Design review of the part built by this model. Coordinates are the model's own, in mm. Coordinates: 2 decimals unless noted, no trailing zeros. Order: outer loops, then holes, each group sorted by start corner. A loop starts at its lowest first (then second) coordinate and runs counter-clockwise, first axis right, second up. Notation, with made-up numbers: M 24.5,-32.75 L 69.5,-32.75 A18 ccw 69.5,-27.75 Z; hole C -35.5,11 d3. An arc over 180 degrees is marked long. Answer as a JSON object with one key per item and string values.
Autodesk Inventor part; units mm, degrees
ref_plane "YZ Plane" through (0, 0, 0) normal (1, 0, 0) x (0, 1, 0)
ref_plane "XZ Plane" through (0, 0, 0) normal (0, 1, 0) x (-1, 0, 0)
ref_plane "XY Plane" through (0, 0, 0) normal (0, 0, 1) x (1, 0, 0)
sketch "Sketch1" plane through (0, 0, 0) normal (0, 0, 1) x (1, 0, 0)
  line L0 (-37.6936, 53.8926) -> (212.3064, 53.8926)
  line L1 (212.3064, 53.8926) -> (212.3064, -66.1074)
  line L2 (212.3064, -66.1074) -> (-37.6936, -66.1074)
  line L3 (-37.6936, -66.1074) -> (-37.6936, 53.8926)
  line L4 (12.3064, -66.1074) -> (162.3064, -66.1074)
  line L5 (162.3064, -66.1074) -> (162.3064, 3.8926)
  line L6 (162.3064, 3.8926) -> (12.3064, 3.8926)
  line L7 (12.3064, 3.8926) -> (12.3064, -66.1074)
  line L8 (-37.6936, 53.8926) -> (-34.6936, 53.8926)
  line L9 (-34.6936, 53.8926) -> (-34.6936, 33.8926)
  line L10 (-34.6936, 33.8926) -> (-37.6936, 33.8926)
  line L11 (-37.6936, 33.8926) -> (-37.6936, 53.8926)
  line L12 (-37.6936, 33.8926) -> (-34.6936, 33.8926)
  line L13 (-34.6936, 33.8926) -> (-34.6936, 13.9926)
  line L14 (-34.6936, 13.9926) -> (-37.6936, 13.9926)
  line L15 (-37.6936, 13.9926) -> (-37.6936, 33.8926)
  line L16 (-37.6936, 13.9926) -> (-34.6936, 13.9926)
  line L17 (-34.6936, 13.9926) -> (-34.6936, -6.0074)
  line L18 (-34.6936, -6.0074) -> (-37.6936, -6.0074)
  line L19 (-37.6936, -6.0074) -> (-37.6936, 13.9926)
  line L20 (-34.6936, -6.0074) -> (-37.6936, -6.0074)
  line L21 (-37.6936, -6.0074) -> (-37.6936, -25.9074)
  line L22 (-37.6936, -25.9074) -> (-34.6936, -25.9074)
  line L23 (-34.6936, -25.9074) -> (-34.6936, -6.0074)
  line L24 (-37.6936, -25.9074) -> (-34.6936, -25.9074)
  line L25 (-34.6936, -25.9074) -> (-34.6936, -45.9074)
  line L26 (-34.6936, -45.9074) -> (-37.6936, -45.9074)
  line L27 (-37.6936, -45.9074) -> (-37.6936, -25.9074)
  line L28 (-34.6936, -45.9074) -> (-37.6936, -45.9074)
  line L29 (-37.6936, -45.9074) -> (-37.6936, -66.1074)
  line L30 (-37.6936, -66.1074) -> (-34.6936, -66.1074)
  line L31 (-34.6936, -66.1074) -> (-34.6936, -45.9074)
  line L32 (212.3064, -66.1074) -> (212.3064, 53.8926)
  line L33 (212.3064, 53.8926) -> (209.3064, 53.8926)
  line L34 (209.3064, 53.8926) -> (209.3064, 33.8926)
  line L35 (209.3064, 33.8926) -> (212.3064, 33.8926)
  line L36 (212.3064, 33.8926) -> (212.3064, 53.8926)
  line L37 (212.3064, 33.8926) -> (209.3064, 33.8926)
  line L38 (209.3064, 33.8926) -> (209.3064, 13.9926)
  line L39 (209.3064, 13.9926) -> (212.3064, 13.9926)
  line L40 (212.3064, 13.9926) -> (212.3064, 33.8926)
  line L41 (212.3064, 13.9926) -> (209.3064, 13.9926)
  line L42 (209.3064, 13.9926) -> (209.3064, -6.0074)
  line L43 (209.3064, -6.0074) -> (212.3064, -6.0074)
  line L44 (212.3064, -6.0074) -> (212.3064, 13.9926)
  line L45 (209.3064, -6.0074) -> (212.3064, -6.0074)
  line L46 (212.3064, -6.0074) -> (212.3064, -25.9074)
  line L47 (212.3064, -25.9074) -> (209.3064, -25.9074)
  line L48 (209.3064, -25.9074) -> (209.3064, -6.0074)
  line L49 (212.3064, -25.9074) -> (209.3064, -25.9074)
  line L50 (209.3064, -25.9074) -> (209.3064, -45.9074)
  line L51 (209.3064, -45.9074) -> (212.3064, -45.9074)
  line L52 (212.3064, -45.9074) -> (212.3064, -25.9074)
  line L53 (209.3064, -45.9074) -> (212.3064, -45.9074)
  line L54 (212.3064, -45.9074) -> (212.3064, -66.1074)
  line L55 (212.3064, -66.1074) -> (209.3064, -66.1074)
  line L56 (209.3064, -66.1074) -> (209.3064, -45.9074)
  line L57 (-34.6936, 53.8926) -> (-14.7936, 53.8926)
  line L58 (-14.7936, 53.8926) -> (-14.7936, 50.8926)
  line L59 (-14.7936, 50.8926) -> (-34.6936, 50.8926)
  line L60 (-34.6936, 50.8926) -> (-34.6936, 53.8926)
  line L61 (-14.7936, 50.8926) -> (5.2064, 50.8926)
  line L62 (5.2064, 50.8926) -> (5.2064, 53.8926)
  line L63 (5.2064, 53.8926) -> (-14.7936, 53.8926)
  line L64 (-14.7936, 53.8926) -> (-14.7936, 50.8926)
  line L65 (5.2064, 50.8926) -> (25.1064, 50.8926)
  line L66 (25.1064, 50.8926) -> (25.1064, 53.8926)
  line L67 (25.1064, 53.8926) -> (5.2064, 53.8926)
  line L68 (5.2064, 53.8926) -> (5.2064, 50.8926)
  line L69 (25.1064, 50.8926) -> (45.1064, 50.8926)
  line L70 (45.1064, 50.8926) -> (45.1064, 53.8926)
  line L71 (45.1064, 53.8926) -> (25.1064, 53.8926)
  line L72 (25.1064, 53.8926) -> (25.1064, 50.8926)
  line L73 (45.1064, 50.8926) -> (65.0064, 50.8926)
  line L74 (65.0064, 50.8926) -> (65.0064, 53.8926)
  line L75 (65.0064, 53.8926) -> (45.1064, 53.8926)
  line L76 (45.1064, 53.8926) -> (45.1064, 50.8926)
  line L77 (65.0064, 50.8926) -> (85.0064, 50.8926)
  line L78 (85.0064, 50.8926) -> (85.0064, 53.8926)
  line L79 (85.0064, 53.8926) -> (65.0064, 53.8926)
  line L80 (65.0064, 53.8926) -> (65.0064, 50.8926)
  line L81 (85.0064, 50.8926) -> (104.9064, 50.8926)
  line L82 (104.9064, 50.8926) -> (104.9064, 53.8926)
  line L83 (104.9064, 53.8926) -> (85.0064, 53.8926)
  line L84 (85.0064, 53.8926) -> (85.0064, 50.8926)
  line L85 (104.9064, 50.8926) -> (124.9064, 50.8926)
  line L86 (124.9064, 50.8926) -> (124.9064, 53.8926)
  line L87 (124.9064, 53.8926) -> (104.9064, 53.8926)
  line L88 (104.9064, 53.8926) -> (104.9064, 50.8926)
  line L89 (124.9064, 50.8926) -> (144.8064, 50.8926)
  line L90 (144.8064, 50.8926) -> (144.8064, 53.8926)
  line L91 (144.8064, 53.8926) -> (124.9064, 53.8926)
  line L92 (124.9064, 53.8926) -> (124.9064, 50.8926)
  line L93 (144.8064, 50.8926) -> (164.8064, 50.8926)
  line L94 (164.8064, 50.8926) -> (164.8064, 53.8926)
  line L95 (164.8064, 53.8926) -> (144.8064, 53.8926)
  line L96 (144.8064, 53.8926) -> (144.8064, 50.8926)
  line L97 (164.8064, 50.8926) -> (184.7064, 50.8926)
  line L98 (184.7064, 50.8926) -> (184.7064, 53.8926)
  line L99 (184.7064, 53.8926) -> (164.8064, 53.8926)
  line L100 (164.8064, 53.8926) -> (164.8064, 50.8926)
  line L101 (184.7064, 50.8926) -> (209.3064, 50.8926)
  line L102 (209.3064, 50.8926) -> (209.3064, 53.8926)
  line L103 (209.3064, 53.8926) -> (184.7064, 53.8926)
  line L104 (184.7064, 53.8926) -> (184.7064, 50.8926)
  point P0 (0, 0)
  point P1 (212.3064, -45.9074)
  point P2 (212.3064, -25.9074)
  point P3 (212.3064, -6.0074)
  point P4 (212.3064, 13.9926)
  point P5 (212.3064, 33.8926)
  point P6 (-37.6936, 13.9926)
  point P7 (-14.7936, 53.8926)
  point P8 (-34.6936, 50.8926)
  point P9 (209.3064, 53.8926)
  point P10 (212.3064, 13.9926)
  point P11 (212.3064, 23.9426)
  point P12 (209.3064, 23.9426)
  point P13 (212.3064, -15.9574)
  point P14 (209.3064, -15.9574)
  dimension "d0" = 250
  dimension "d1" = 120
  dimension "d14" = 150
  dimension "d15" = 70
  dimension "d16" = 50
  dimension "d17" = 3
  dimension "d18" = 20
  dimension "d19" = 19.9
  dimension "d20" = 20
  dimension "d21" = 19.9
  dimension "d22" = 20
  dimension "d25" = 19.9
  dimension "d26" = 3
  dimension "d27" = 20
  dimension "d28" = 19.9
  dimension "d29" = 20
  dimension "d30" = 19.9
  dimension "d31" = 20
  dimension "d32" = 19.9
  dimension "d33" = 20
  dimension "d34" = 19.9
  dimension "d35" = 20
  dimension "d36" = 19.9
  dimension "d37" = 3
  dimension "d38" = 3
extrude "Extrusion1" add sketch "Sketch1" along normal blind 3 contours L0 L9 L10 L3 | L0 L62 L61 L58 | L59 L61 L65 L69 L73 L77 L81 L85 L89 L93 L97 L101 L34 L38 L42 L48 L50 L56 L2 L5 L6 L7 L31 L25 L23 L17 L13 L9 | L14 L17 L18 L3 | L0 L70 L69 L66 | L22 L25 L26 L3 | L0 L78 L77 L74 | L0 L86 L85 L82 | L0 L94 L93 L90 | L50 L47 L1 L51 | L0 L34 L101 L98 | L0 L1 L35 L34 | L42 L39 L1 L43
equation "\"d16\" = -0.5 * d14 + 0.5 * d0"
equation "\"d19\" = d25"
equation "\"d21\" = d25"
equation "\"d28\" = d25"
equation "\"d30\" = d25"
1) To check wall thickness, follow L1, parallel to X at y = -15.5, z = 1.65; L2, parallel to X at y = -41, z = 2.7; L3, parallel to X at y = 29, z = 2. State the ranges of each line that lie inside material, in increasing order.
Taken from the geometry:
{"L1": "x = -34.69 to 12.31, 162.31 to 209.31", "L2": "x = -37.69 to 12.31, 162.31 to 212.31", "L3": "x = -34.69 to 209.31"}
2) Add section B-B (y = -23.5). State the section outline as (x, z) points.
Taken from the geometry:
{"outline": "M -34.69,0 L 12.31,0 L 12.31,3 L -34.69,3 Z; M 162.31,0 L 209.31,0 L 209.31,3 L 162.31,3 Z"}
3) Insertion check: pin 1 Ø0.9 at (x, z) = (-25, 1.5) entering from +Y; pin 2 Ø1.5 at (x, z) = (-36.5, 1) entering from -Y; pin 3 Ø1.5 at (y, z) = (-13, 1.5) entering from -X. Each pin has a flat end and moves straight along its axis. Give the tip position at first contact, or say it passes through.
Taken from the geometry:
{"pin 1": "stops at y = 50.89", "pin 2": "stops at y = -45.91", "pin 3": "stops at x = -34.69"}
4) Add section D-D (y = 23). State the section outline as (x, z) points.
Taken from the geometry:
{"outline": "M -34.69,0 L 209.31,0 L 209.31,3 L -34.69,3 Z"}
5) Add section C-C (x = 51). State the section outline as (y, z) points, and give its area (3 significant figures).
Taken from the geometry:
{"outline": "M 3.89,0 L 50.89,0 L 50.89,3 L 3.89,3 Z", "area": "141 mm2"}
6) Add section A-A (y = -39). State the section outline as (x, z) points, and give its area (3 significant figures).
Taken from the geometry:
{"outline": "M -37.69,0 L 12.31,0 L 12.31,3 L -37.69,3 Z; M 162.31,0 L 212.31,0 L 212.31,3 L 162.31,3 Z", "area": "300 mm2"}
